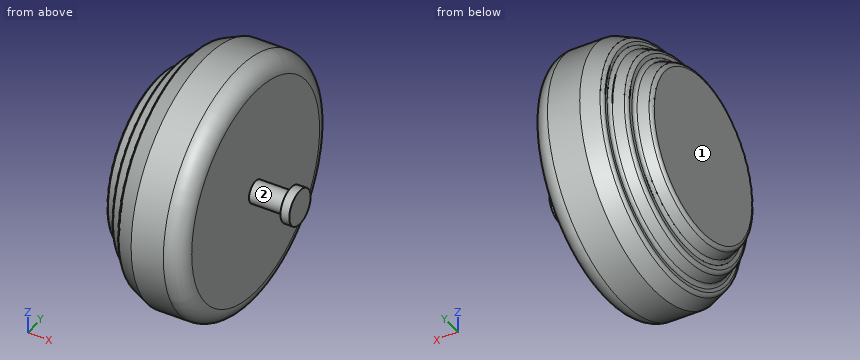
```python
from build123d import *

# Parameters (mm, degrees)
REDONDEO3_R             = 5
CROQUIS2_R              = 12.5
SALIENTE_EXTRUIR1_DEPTH = 40
CROQUIS3_R              = 20
SALIENTE_EXTRUIR2_DEPTH = 10


with BuildPart() as part:
    # Croquis1 → Revoluci_n1 (revolve)
    with BuildSketch(Plane(origin=(0, 0, 0), x_dir=(1, 0, 0), z_dir=(0, 1, 0)), mode=Mode.PRIVATE) as revoluci_n1_sk:
        with BuildLine():
            Line((106.445710743, 140), (70.03994637, 140))
            Line((70.03994637, 140), (48.737618848, 130.932753785))
            Line((48.737618848, 130.932753785), (48.737618848, 120.610275725))
            Line((48.737618848, 120.610275725), (31.868809424, 113.430137863))
            Line((31.868809424, 113.430137863), (31.868809424, 102.180137863))
            Line((31.868809424, 102.180137863), (15, 95))
            Line((15, 95), (15, 0))
            Line((15, 0), (70, 0))
            Line((70, 0), (126.445710743, 0))
            Line((126.445710743, 0), (126.445710743, 120))
            ThreePointArc((126.445710743, 120), (120.587846367, 134.142135624), (106.445710743, 140))
        make_face()
    revolve(revoluci_n1_sk.sketch.rotate(Axis((-209.218950064, 0, 0), (1, 0, 0)), 180), axis=Axis((-209.218950064, 0, 0), (1, 0, 0)))

    # Redondeo3
    redondeo3_edges = [part.edges().sort_by_distance(p)[0] for p in [
        (15, 0, -95),
        (31.868809424, 0, -102.180137863),
        (31.868809424, 0, -113.430137863),
        (48.737618848, 0, -120.610275725),
        (48.737618848, 0, -130.932753785),
    ]]
    fillet(redondeo3_edges, radius=REDONDEO3_R)

    # Croquis2 → Saliente-Extruir1 (add)
    with BuildSketch(Plane(origin=(126.445710743, 0, 0), x_dir=(0, 0, -1), z_dir=(1, 0, 0))):
        Circle(CROQUIS2_R)
    extrude(amount=SALIENTE_EXTRUIR1_DEPTH)

    # Croquis3 → Saliente-Extruir2 (add)
    with BuildSketch(Plane(origin=(166.445710743, 0, 0), x_dir=(0, 0, -1), z_dir=(1, 0, 0))):
        Circle(CROQUIS3_R)
    extrude(amount=SALIENTE_EXTRUIR2_DEPTH)


solid = part.part
```
Check sheet for the modelled part. Datum: model origin and axes. Units: mm. Face numbers are marked on the shaded views. A direction names the side the tool comes from. Round coordinates to 2 decimals unless told otherwise and drop trailing zeros. Order: outer loops, then holes, each group sorted by start corner. A loop starts at its lowest first (then second) coordinate and runs counter-clockwise, first axis right, second up. Notation, with made-up numbers: (78.25, 71.25) -> (133.25, 71.25) arc R13 ccw to (133.25, 96.25) -> close; hole circle Ø9 at (-5, 19). An arc over 180 degrees is marked (long way). One line per item, written item: value. Start each with the question number.
Q1. Cross-section at C-C (x = 100). Record the boundary of the cut face in (y, z), and give its area (3 significant figures).
Q2. Set-up check for the marked faces 1 and 2: record each of +Z, -Z, +X, -X, +Y, -Y from which the full face is reachable in a straight line by a thin tool's end or side.
Q3. Cross-section at D-D (x = 144). Record the boundary of the cut face in (y, z), and give its area (3 significant figures).
Q4. Gauge pin test, flat ends, axial feed: pin 1 Ø1.5 at (x, z) = (93.5, 110) entering from +Y; pin 2 Ø1 at (x, z) = (112.5, -59) entering from +Y; pin 3 Ø8 at (x, z) = (108.5, 14) entering from -Y. Record the tip position at first contact, or that the pin passes through.
Q5. Thickness scan on line 1 (X direction, y = -93, z = -50.5); line 2 (X direction, y = -45.5, z = 12); line 3 (Y direction, x = 110, z = -42). Record the ranges inside material, lowest first.
Completed:
1. outline: circle Ø280 at (0, 0)
1. area: 61,600 mm²
2. face 1: +Z, -Z, -X, +Y, -Y
2. face 2: none
3. outline: circle Ø25 at (0, 0)
3. area: 491 mm²
4. pin 1: stops at y = 87.55
4. pin 2: stops at y = 126.21
4. pin 3: stops at y = -139.61
5. line 1: x = 31.87 to 126.45
5. line 2: x = 15 to 126.45
5. line 3: y = -133.22 to 133.22
